Autodesk Inventor part; units mm, degrees
ref_plane "YZ Plane" through (0, 0, 0) normal (1, 0, 0) x (0, 1, 0)
ref_plane "XZ Plane" through (0, 0, 0) normal (0, 1, 0) x (-1, 0, 0)
ref_plane "XY Plane" through (0, 0, 0) normal (0, 0, 1) x (1, 0, 0)
sketch "Skizze1" plane through (0, 0, 0) normal (0, 0, 1) x (1, 0, 0)
  line L0 (0, 5.6) -> (0, -5.6) construction
  line L1 (-9.1, 0) -> (26.6, 0) construction
  circle A0 centre (0, 0) radius 2
  circle A1 centre (9.5, 0) radius 1
  circle A2 centre (16, 0) radius 1
  circle A3 centre (19, 0) radius 1
  arc A4 (19.1974, -2.4922) -> (19.1974, 2.4922) centre (19, 0) ccw
  arc A5 (0.3158, 3.9875) -> (0.3158, -3.9875) centre (0, 0) ccw
  line L2 (0.3158, 3.9875) -> (19.1974, 2.4922)
  line L3 (0.3158, -3.9875) -> (19.1974, -2.4922)
  circle A6 centre (12.8, 0) radius 1
  circle A7 centre (0, 0) radius 4
  point P0 (0.5263, 3.9652)
  point P1 (0.6579, -1.8887)
  point P2 (0.6579, 1.8887)
  dimension "d0" = 9.5
  dimension "d1" = 16
  dimension "d2" = 19
  dimension "d3" = 5
  dimension "d4" = 2
  dimension "d5" = 4
  dimension "d6" = 8
  dimension "d17" = 12.8
extrude "Extrusion1" add sketch "Skizze1" along normal blind 1.8
extrude "Extrusion2" add sketch "Skizze1" along normal blind 4.5 contours A5 A7
properties part number "Servo-Arm-20mm"
Geometry check sheet. Reference: the model listing, model coordinates, mm. A direction names the side the tool comes from. Coordinates: 2 decimals unless noted, no trailing zeros. Loops run counter-clockwise (first coordinate to the right, second up) from the corner with the lowest first, then second, coordinate; pieces in that order, holes last.
Item 1: Sectioned sample at D-D, the plane x = 9.5. Record the boundary of the cut face in (y, z), then the cut area to 3 significant figures.
Item 2: Sectioned sample at A-A, the plane z = 1.3. Record the boundary of the cut face in (x, y).
Item 3: Thickness scan on line 1 (Y direction, x = 0, z = 2.45); line 2 (Z direction, x = 16.75, y = 2.25); line 3 (X direction, y = 1.75, z = 1.4). Record the ranges inside material, lowest first.
Item 4: Go/stop test with flat-tipped pins: pin 1 Ø3 at (x, y) = (12.8, 0) entering from -Z; pin 2 Ø4 at (x, y) = (13, -0.5) entering from +Z; pin 3 Ø1.2 at (x, y) = (16, 0) entering from +Z. Record where each tip stops, or that it passes through.
Item 5: Access from +Z, -Z, +X, -X, +Y, -Y to the whole of each face (thin tool, end or side, straight path). Record for faces 4 (the face through (0, 2, 2)), 5 (the face through (4, 0, 3)).
Item 6: Release check for a two-part mould opening along Y. For faces 1 (the face through (13.754, -0.3, 0.887)), 2 (the face through (-4, 0, 2)), 3 (the face through (8.6, -0.8, 0)) record: released by +Y, released by -Y, zero draft, split by the parting line, or undercut.
Item 7: Sectioned sample at C-C, the plane y = 1.5. Record the boundary of the cut face in (x, z), then the cut area to 3 significant figures.
Item 8: Sectioned sample at B-B, the plane x = 0. Record the boundary of the cut face in (y, z).
Check result:
1. outline: (-3.26, 0) - (-1, 0) - (-1, 1.8) - (-3.26, 1.8) - close; (1, 0) - (3.26, 0) - (3.26, 1.8) - (1, 1.8) - close
1. area: 8.14 mm2
2. outline: (0.32, -3.99) - (19.2, -2.49) arc R2.5 ccw to (19.2, 2.49) - (0.32, 3.99) arc R4 ccw (long way) to start; hole circle Ø4 at (0, 0); hole circle Ø2 at (9.5, 0); hole circle Ø2 at (12.8, 0); hole circle Ø2 at (16, 0); hole circle Ø2 at (19, 0)
3. line 1: y = -4 to -2, 2 to 4
3. line 2: z = 0 to 1.8
3. line 3: x = -3.6 to -0.97, 0.97 to 20.79
4. pin 1: stops at z = 0
4. pin 2: stops at z = 1.8
4. pin 3: passes through
5. face 4: +Z, -Z
5. face 5: +Z, +X
6. face 1: undercut
6. face 2: split by the parting line
6. face 3: zero draft
7. outline: (-3.71, 0) - (-1.32, 0) - (-1.32, 4.5) - (-3.71, 4.5) - close; (1.32, 0) - (21, 0) - (21, 1.8) - (3.71, 1.8) - (3.71, 4.5) - (1.32, 4.5) - close
7. area: 52.6 mm2
8. outline: (-4, 0) - (-2, 0) - (-2, 4.5) - (-4, 4.5) - close; (2, 0) - (4, 0) - (4, 4.5) - (2, 4.5) - close
